Read the model definition and answer for the solid it produces. Units are mm, in the model's axes. Face numbers are marked on the shaded views. Coordinates: 2 decimals unless noted, no trailing zeros. Loops run counter-clockwise (first coordinate to the right, second up) from the corner with the lowest first, then second, coordinate; pieces in that order, holes last. Notation, with made-up numbers: (-9.75, 81) -> (36.25, 81) arc R35 ccw to (36.25, 116) -> close; hole circle Ø9 at (61.5, 0.25). An arc over 180 degrees is marked (long way). Answer as a JSON object with one key per item and string values. Group by question number.
Q1. Determine the mould class of the marked faces 1, 2, 3 and 4 for opening direction Z: released by +Z, released by -Z, zero draft, split by the parting line, or undercut.
Q2. The part is cut by section D-D on y = 3.5. Write down the section's boundary in (x, z) (3 decimals), and give its area (3 significant figures).
Q3. Straight lines are drawn through the part: line 1 along X through (y, z) = (5.5, 0) (3 decimals); line 2 along Z through (x, y) = (-11.5, 15.5); line 3 along Y through (x, z) = (-3.5, -22). For each, find the intervals that lie inside material, in ascending order. Write a range as [from, to].
Q4. The part is cut by section B-B on y = 28. Write down the section's boundary in (x, z).
Q5. Each of these flat-tipped pins is pushed along its axis until it touches: P1, Ø0.9, axis at x = -24, z = 4.5, coming from the +Y side; P2, Ø12, axis at x = 3.5, y = 20, coming from the -Z side; P3, Ø8, axis at y = 13, z = -34, coming from the +X side. Where does it stop, or does it pass through?
from build123d import *

# Parameters (mm, degrees)
SKETCH1_W            = 50.975
SKETCH1_H            = 38.1
BASE_DEPTH           = 7.9375
SKETCH2_R            = 11
BEARING_BORE_DEPTH   = 7
THRU_HOLE_DEPTH      = 36.191831439
THRU_HOLE_DEPTH_BACK = 36.191831439
SKETCH3_R            = 9.525
SKETCH4_W            = 7.9375
SKETCH4_H            = 38.1
VERTICAL_DEPTH       = 25.4
SKETCH7_W            = 6.35
SKETCH7_H            = 25.4
ARM_STOP_DEPTH       = 20.8026
ANGLED_FACE_REACH    = 49.967
FILLET1_R            = 7.62
SKETCH6_R            = 1.5
DOWEL_HOLES_DEPTH    = 7.007999954
SPRING_BASE_DEPTH    = 25.4
SKETCH12_R           = 2.794
SPRING_MOUNT_DEPTH   = 25.4


with BuildPart() as part:
    # Sketch1 → Base (new body)
    with BuildSketch(Plane(origin=(0, 0, 0), x_dir=(1, 0, 0), z_dir=(0, 1, 0))):
        with Locations((-3.2625, 0)):
            Rectangle(SKETCH1_W, SKETCH1_H)
    extrude(amount=BASE_DEPTH)

    # Sketch2 → Bearing Bore (cut)
    with BuildSketch(Plane(origin=(0, 7.9375, 0), x_dir=(1, 0, 0), z_dir=(0, 1, 0))):
        with Locations(Location((0, 0, 0), (0, 0, 270))):
            Circle(SKETCH2_R)
    extrude(amount=-BEARING_BORE_DEPTH, mode=Mode.SUBTRACT)

    # Sketch3 → Thru Hole (cut, two sides: drawn at the far end of the back side and taken through both)
    with BuildSketch(Plane(origin=(0, 0.9375, 0), x_dir=(1, 0, 0), z_dir=(0, 1, 0)).offset(-THRU_HOLE_DEPTH_BACK)):
        with Locations(Location((0, 0, 0), (0, 0, 270))):
            Circle(SKETCH3_R)
    extrude(amount=THRU_HOLE_DEPTH + THRU_HOLE_DEPTH_BACK, mode=Mode.SUBTRACT)

    # Sketch4 → Vertical (add)
    with BuildSketch(Plane(origin=(0, 7.9375, 0), x_dir=(1, 0, 0), z_dir=(0, 1, 0))):
        with Locations((-24.78125, 0)):
            Rectangle(SKETCH4_W, SKETCH4_H)
    extrude(amount=VERTICAL_DEPTH)

    # Sketch7 → Arm Stop (add)
    with BuildSketch(Plane(origin=(-20.8125, 0, 0), x_dir=(0, 0, -1), z_dir=(1, 0, 0))):
        with Locations((-15.875, 20.6375)):
            Rectangle(SKETCH7_W, SKETCH7_H)
    extrude(amount=ARM_STOP_DEPTH)

    # Sketch8 → Angled Face (add, up to next)
    with BuildSketch(Plane(origin=(0, 33.3375, 0), x_dir=(1, 0, 0), z_dir=(0, 1, 0)), mode=Mode.PRIVATE) as angled_face_sk1:
        Polygon((-0.0099, -12.7), (5.318382658, -19.05), (-0.0099, -19.05), align=None)
    angled_face_tool1 = extrude(angled_face_sk1.sketch, amount=-ANGLED_FACE_REACH, mode=Mode.PRIVATE) - part.part
    add(angled_face_tool1.solids().sort_by_distance((1.766194, 33.3375, 16.933333))[0])

    # Fillet1
    fillet1_edges = [part.edges().sort_by_distance(p)[0] for p in [
        (-20.8125, 20.6375, 12.7),
    ]]
    fillet(fillet1_edges, radius=FILLET1_R)

    # Sketch6 → Dowel Holes (cut)
    with BuildSketch(Plane(origin=(0, 33.3375, 0), x_dir=(1, 0, 0), z_dir=(0, 1, 0))):
        with Locations(Location((-24.78125, 14.990388599, 0), (0, 0, 270))):
            Circle(SKETCH6_R)
        with Locations(Location((-24.78125, 4.9967962, 0), (0, 0, 270))):
            Circle(SKETCH6_R)
        with Locations(Location((-24.78125, -14.990388599, 0), (0, 0, 270))):
            Circle(SKETCH6_R)
        with Locations(Location((-24.78125, -4.9967962, 0), (0, 0, 270))):
            Circle(SKETCH6_R)
    extrude(amount=-DOWEL_HOLES_DEPTH, mode=Mode.SUBTRACT)

    # Sketch11 → Spring Base (add)
    with BuildSketch(Plane(origin=(0, 0, -19.05), x_dir=(-1, 0, 0), z_dir=(0, 0, -1))):
        Polygon((-22.225, 7.9375), (20.8125, 7.9375), (20.8125, 33.3375), (28.75, 33.3375), (28.75, 0), (-22.225, 0), align=None)
    extrude(amount=SPRING_BASE_DEPTH)

    # Sketch12 → Spring Mount (add)
    with BuildSketch(Plane(origin=(0, 7.9375, 0), x_dir=(1, 0, 0), z_dir=(0, 1, 0))):
        with Locations(Location((-16.7612, 31.75, 0), (0, 0, 270))):
            Circle(SKETCH12_R)
    extrude(amount=SPRING_MOUNT_DEPTH)


solid = part.part
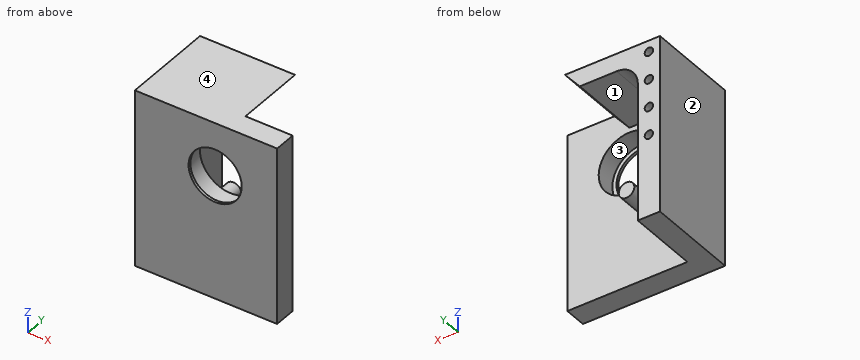
Final values:
{
 "1": {"face 1": "released by -Z", "face 2": "zero draft", "face 3": "undercut", "face 4": "released by +Z"},
 "2": {"outline": "(-28.75, -44.45) -> (22.225, -44.45) -> (22.225, 19.05) -> (-28.75, 19.05) -> close; hole circle Ø22 at (0, 0)", "area": "2,860 mm2"},
 "3": {"line 1": "x = [-28.75, -11], [11, 22.225]", "line 2": "z = [12.7, 19.05]", "line 3": "y = [0, 7.94]"},
 "4": {"outline": "(-28.75, -44.45) -> (-20.81, -44.45) -> (-20.81, 5.08) arc R7.62 cw to (-13.19, 12.7) -> (-0.01, 12.7) -> (5.32, 19.05) -> (-28.75, 19.05) -> close; circle Ø5.59 at (-16.76, -31.75); hole circle Ø3 at (-24.78, -14.99); hole circle Ø3 at (-24.78, -5); hole circle Ø3 at (-24.78, 5); hole circle Ø3 at (-24.78, 14.99)"},
 "5": {"P1": "stops at y = 26.33", "P2": "stops at z = 12.7", "P3": "stops at x = -13.97"}
}
